```python
from build123d import *

# Parameters (mm, degrees)
F1_DEPTH = 60.325
F2_R     = 7.9375
F2_R_2   = 2.38125
F3_DEPTH = 4.9359792052


with BuildPart() as f1:
    # F0 (on Right) → F1 (new body, symmetric)
    with BuildSketch(Plane.YZ):
        with BuildLine():
            Line((0, 0), (0, 6.35))
            Line((0, 6.35), (-50.8, 6.35))
            Line((-50.8, 6.35), (-50.8, 4.8701947642))
            ThreePointArc((-50.8, 4.8701947642), (-25.322261732, 3.2459692683), (0, 0))
        make_face()
    extrude(amount=F1_DEPTH, both=True)

    # F2 (on face) → F3 (cut, up to face)
    with BuildSketch(Plane.XY.offset(6.35)):
        with Locations((0, -25.4)):
            Circle(F2_R)
        with Locations((-22.225, -25.4)):
            Circle(F2_R_2)
        with Locations((22.225, -25.4)):
            Circle(F2_R_2)
    extrude(amount=-F3_DEPTH, mode=Mode.SUBTRACT)


solid = f1.part
```
CAD build for the part. Positions are in the model's coordinates, mm. Round coordinates to 2 decimals unless told otherwise and drop trailing zeros. Order: outer loops, then holes, each group sorted by start corner. A loop starts at its lowest first (then second) coordinate and runs counter-clockwise, first axis right, second up.
Item 1: Mould opens along X. For faces 1 (the face through (23.505, -23.392, 4.708)), 2 (the face through (-60.325, -20, 5)), 3 (the face through (60.325, -20, 5)), 4 (the face through (-1.03, -17.53, 4.85)) say: pulls with the +X half, pulls with the -X half, needs draft (parallel to the pull), parting line crosses it, or undercut.
Item 2: Pin check, flat tips, straight feed: pin 1 (4 mm diameter, centred on x = -22.225, y = -25.4, fed in from -Z); pin 2 (6 mm diameter, centred on x = -24.5, y = -20, fed in from -Z). Stop position of each tip, or through.
Item 3: Probe line 1 along X through (y, z) = (-25.4, 3.6) (1 decimal); line 2 along Z through (x, y) = (-21.5, -17.5); line 3 along Z through (x, y) = (-4, -10). List the from-to ranges inside material, lowest first.
Item 4: Saw through at B-B on x = 0. Write the cut outline in (y, z), then the cut area to 3 significant figures.
Item 5: Saw through at C-C on x = 39. Write the cut outline in (y, z).
Item 6: Saw through at A-A on y = -29.5. Write the cut outline in (x, z) (3 decimals), then the cut area to 3 significant figures.
Reported:
1. face 1: undercut
1. face 2: pulls with the -X half
1. face 3: pulls with the +X half
1. face 4: undercut
2. pin 1: passes through
2. pin 2: stops at z = 2.36
3. line 1: x = -60.3 to -24.6, -19.8 to -7.9, 7.9 to 19.8, 24.6 to 60.3
3. line 2: z = 2.42 to 6.35
3. line 3: z = 1.48 to 6.35
4. outline: (-50.8, 4.87) arc R400.05 cw to (-33.34, 3.93) - (-33.34, 6.35) - (-50.8, 6.35) - close; (-17.46, 2.41) arc R400.05 cw to (0, 0) - (0, 6.35) - (-17.46, 6.35) - close
4. area: 122 mm2
5. outline: (-50.8, 4.87) arc R400.05 cw to (0, 0) - (0, 6.35) - (-50.8, 6.35) - close
6. outline: (-60.325, 3.624) - (-6.797, 3.624) - (-6.797, 6.35) - (-60.325, 6.35) - close; (6.797, 3.624) - (60.325, 3.624) - (60.325, 6.35) - (6.797, 6.35) - close
6. area: 292 mm2
